```python
from build123d import *

# Parameters (mm, degrees)
IZIM1_R                     = 6
IZIM1_R_2                   = 1.5
Y_KSEKLIK_EKSTR_ZYON1_DEPTH = 2
RADYUS1_R                   = 8
IZIM5_R                     = 35.5
Y_KSEKLIK_EKSTR_ZYON2_DEPTH = 1
IZIM6_R                     = 2
Y_KSEKLIK_EKSTR_ZYON3_DEPTH = 20
IZIM7_R                     = 4
Y_KSEKLIK_EKSTR_ZYON4_DEPTH = 2
Y_KSEKLIK_EKSTR_ZYON5_DEPTH = 24
Y_KSEKLIK_EKSTR_ZYON6_DEPTH = 3


with BuildPart() as part:
    # Çizim1 → Yükseklik-Ekstrüzyon1 (new body)
    with BuildSketch(Plane.XY):
        with BuildLine():
            Line((8, 27.5), (8, 8))
            Line((8, 8), (27.5, 8))
            ThreePointArc((27.5, 8), (35.5, 0), (27.5, -8))
            Line((27.5, -8), (8, -8))
            Line((8, -8), (8, -27.5))
            ThreePointArc((8, -27.5), (0, -35.5), (-8, -27.5))
            Line((-8, -27.5), (-8, -8))
            Line((-8, -8), (-27.5, -8))
            ThreePointArc((-27.5, -8), (-35.5, 0), (-27.5, 8))
            Line((-27.5, 8), (-8, 8))
            Line((-8, 8), (-8, 27.5))
            ThreePointArc((-8, 27.5), (0, 35.5), (8, 27.5))
        make_face()
        Circle(IZIM1_R, mode=Mode.SUBTRACT)
        with Locations((0, 9.5)):
            Circle(IZIM1_R_2, mode=Mode.SUBTRACT)
        with Locations((0, -9.5)):
            Circle(IZIM1_R_2, mode=Mode.SUBTRACT)
        with Locations((-12.5, 0)):
            Circle(IZIM1_R_2, mode=Mode.SUBTRACT)
        with Locations((12.5, 0)):
            Circle(IZIM1_R_2, mode=Mode.SUBTRACT)
        with Locations((0, 27.5)):
            Circle(IZIM1_R_2, mode=Mode.SUBTRACT)
        with Locations((27.5, 0)):
            Circle(IZIM1_R_2, mode=Mode.SUBTRACT)
        with Locations((0, -27.5)):
            Circle(IZIM1_R_2, mode=Mode.SUBTRACT)
        with Locations((-27.5, 0)):
            Circle(IZIM1_R_2, mode=Mode.SUBTRACT)
    extrude(amount=Y_KSEKLIK_EKSTR_ZYON1_DEPTH)

    # Radyus1
    radyus1_edges = [part.edges().sort_by_distance(p)[0] for p in [
        (8, 8, 1),
        (8, -8, 1),
        (-8, -8, 1),
        (-8, 8, 1),
    ]]
    fillet(radyus1_edges, radius=RADYUS1_R)

    # Çizim4 → Döndür1 (revolve)
    with BuildSketch(Plane(origin=(0, 0, 0), x_dir=(0, 0, -1), z_dir=(1, 0, 0))):
        Polygon((0, 27.5), (0, 35.5), (8, 43.5), (52, 43.5), (60, 35.5), (60, 27.5), (52, 35.5), (52, 31.5), (53.414213562, 30.085786438), (53.414213562, 0), (6.585786438, 0), (6.585786438, 30.085786438), (8, 31.5), (8, 35.5), align=None)
    revolve(axis=Axis((0, 0, -6.585786438), (0, 0, -1)))

    # Çizim5 → Yükseklik-Ekstrüzyon2 (add)
    with BuildSketch(Plane(origin=(0, 0, -60), x_dir=(-1, 0, 0), z_dir=(0, 0, -1))):
        Circle(IZIM5_R)
    extrude(amount=Y_KSEKLIK_EKSTR_ZYON2_DEPTH)

    # Çizim6 → Yükseklik-Ekstrüzyon3 (add)
    with BuildSketch(Plane.XY.offset(-6.585786438)):
        Circle(IZIM6_R)
    extrude(amount=Y_KSEKLIK_EKSTR_ZYON3_DEPTH)

    # Çizim7 → Yükseklik-Ekstrüzyon4 (add)
    with BuildSketch(Plane.XY.offset(13.414213562)):
        Circle(IZIM7_R)
    extrude(amount=Y_KSEKLIK_EKSTR_ZYON4_DEPTH)

    # Çizim9 → Yükseklik-Ekstrüzyon5 (add)
    with BuildSketch(Plane.XY.offset(15.414213562)):
        Polygon((4, 0), (2, 3.464101615), (-2, 3.464101615), (-4, 0), (-2, -3.464101615), (2, -3.464101615), align=None)
    extrude(amount=Y_KSEKLIK_EKSTR_ZYON5_DEPTH)

    # Çizim10 → Yükseklik-Ekstrüzyon6 (add)
    with BuildSketch(Plane.XY.offset(39.414213562)):
        Polygon((5.773502692, 0), (2.886751346, 5), (-2.886751346, 5), (-5.773502692, 0), (-2.886751346, -5), (2.886751346, -5), align=None)
    extrude(amount=Y_KSEKLIK_EKSTR_ZYON6_DEPTH)

    # Çizim11 → Döndür2 (revolve)
    with BuildSketch(Plane(origin=(0, 0, 0), x_dir=(0, 0, -1), z_dir=(1, 0, 0))):
        with BuildLine():
            Line((-42.414213562, 0), (-50.414213562, 0))
            ThreePointArc((-50.414213562, 0), (-46.98644571, 3.170331375), (-42.414213562, 4.116527269))
            Line((-42.414213562, 4.116527269), (-42.414213562, 0))
        make_face()
    revolve(axis=Axis((0, 0, 42.414213562), (0, 0, 1)))


solid = part.part
```
Source: CAD feature listing. Evaluate the final solid. Frame: model axes, mm. A direction names the side the tool comes from. Give positions to 0.01 mm unless a question says otherwise; leave off trailing zeros. Write each loop counter-clockwise with the first axis right and the second up, starting at its lowest first coordinate (ties: lowest second). Pieces come first, ordered by that corner, then holes.
1. Material intervals for line 1 along Z through (x, y) = (-2, -8.5); line 2 along Z through (x, y) = (4, -28); line 3 along Z through (x, y) = (18, -10.5), sorted ascending.
2. Access query for faces 1 (the face through (0, -5, 41)), 2 (the face through (0, 3.464, 27)), 3 (the face through (-0.867, -3.905, 14.4)), 4 (the face through (-3.014, -1.708, 27.246)), 5 (the face through (26, 0, 1)). Directions: +Z, -Z, +X, -X, +Y, -Y. A direction counts if a zero-diameter tool reaches every point of the face in a straight line with its end or side. Return the directions, or none.
3. Section query C-C (z = 4). Return the cut outline in (x, y), then the cut area to 3 significant figures.
4. Section query A-A (x = -12.5). Count the separate pieces of the cut face and the enclosed holes in it, then the cut area to 3 significant figures.
5. Pull-direction query (Z, two-part tool) for faces 6 (the face through (20, -22, 0)), 7 (the face through (-29, 0, 1)), 8 (the face through (0, 0, -61)), 9 (the face through (-29, 13, -8)); classes: +Z half, -Z half, draft (parallel to the pull), parting line (faces both ways), or undercut.
6. First-contact query: pin 1 (2.5 mm diameter, centred on x = 1, z = 41, fed in from +Y); pin 2 (2 mm diameter, centred on x = -11.5, y = 27, fed in from +Z); pin 3 (1.5 mm diameter, centred on x = -23.5, z = -45.5, fed in from -Y). Flat tips, straight axial feed; report the tip coordinate or a pass-through.
Output values:
1. line 1: z = -61 to -60, -53.41 to -6.59, 0 to 2
1. line 2: z = -61 to -59.22, -53.41 to -6.59, -0.78 to 2
1. line 3: z = -61 to -60, -53.41 to -6.59
2. face 1: +Z, +X, -X, -Y
2. face 2: +X, -X, +Y
2. face 3: none
2. face 4: -X, -Y
2. face 5: +Z
3. outline: circle Ø4 at (0, 0)
3. area: 12.6 mm2
4. separate pieces: 3
4. enclosed holes: 1
4. area: 4,200 mm2
5. face 6: +Z half
5. face 7: draft
5. face 8: -Z half
5. face 9: undercut
6. pin 1: stops at y = 5
6. pin 2: stops at z = 0
6. pin 3: stops at y = -37.08
